For this review, take the finished solid that the model builds, in its own axes (mm). A direction names the side the tool comes from. Coordinates: 2 decimals unless noted, no trailing zeros. Order: outer loops, then holes, each group sorted by start corner. A loop starts at its lowest first (then second) coordinate and runs counter-clockwise, first axis right, second up. Notation, with made-up numbers: (-16, -15) - (39, -15) arc R33 ccw to (39, 20) - close; hole circle Ø9 at (48, 13.5). An arc over 180 degrees is marked (long way). One line per item, written item: value. Start each with the question number.
(1) Consider section C-C on y = 62. Write out the cut boundary in (x, z) (3 decimals), then the cut area to 3 significant figures.
(2) Consider section D-D on x = 34. Write out the cut boundary in (y, z).
(3) For faces 1 (the cylindrical face through (18.37, 87.68, 11.06)), 2 (the flat face through (10, 0, 7)), list the 3-axis set-ups (+Z, -Z, +X, -X, +Y, -Y) from which the entire face can be reached by the end or side of a thin tool; tool diameter is ignored.
(4) Consider section A-A on z = 5. Write out the cut boundary in (x, y).
(5) To check wall thickness, follow line 1 along Y through (x, z) = (55, 5.75); line 2 along Y through (x, z) = (130, 1.5); line 3 along X through (y, z) = (100, 10.5). State the ranges of each line that lie inside material, in increasing order.
(6) Consider section B-B on x = 130. Write out the cut boundary in (y, z).
(7) Clearance check with flat-ended pins moving along their axes: pin 1 (4.5 mm diameter, centred on x = 17, y = 97, fed in from +Z); pin 2 (8 mm diameter, centred on y = 38.5, z = 12, fed in from +X); pin 3 (14 mm diameter, centred on x = 93, y = 100, fed in from +Z); pin 4 (2 mm diameter, centred on x = 67, z = 2, fed in from -Y). State where each tip first meets the part, or that it passes through.
(8) Mouldability with a two-part tool opening along X and no side actions: class faces 3 (the flat face through (61, 113, 0)), 4 (the flat face through (88, 68, 7)), 5 (the flat face through (0, 75, 7)), 6 (the flat face through (25, 95, 7)) as released by +X, released by -X, zero draft, split by the parting line, or undercut.
```python
from build123d import *

# Parameters (mm, degrees)
EXTRUDE_1_DEPTH               = 15
HOLE_WIZARD_M20_1_D           = 17.5
HOLE_WIZARD_M20_1_CSINK_D     = 20.05
HOLE_WIZARD_M20_1_CSINK_ANGLE = 90
SKETCH_5_R                    = 4.5
CUT_EXTRUDE_1_DEPTH           = 220.715725427
SKETCH_6_R                    = 7.5
CUT_EXTRUDE_2_DEPTH           = 8


with BuildPart() as part:
    # 스케치1 → 보스-돌출1 (new body)
    with BuildSketch(Plane.XY):
        Polygon((155, 135), (20, 0), (0, 0), (0, 152), (3, 155), (155, 155), align=None)
    extrude(amount=EXTRUDE_1_DEPTH)

    # M20 나사 구멍1 (through all)
    with Locations(Plane.XY.offset(15)):
        with Locations((62, 93), (55, 62), (93, 100)):
            CounterSinkHole(HOLE_WIZARD_M20_1_D / 2, HOLE_WIZARD_M20_1_CSINK_D / 2, counter_sink_angle=HOLE_WIZARD_M20_1_CSINK_ANGLE)

    # 스케치5 → 컷-돌출1 (cut, through all)
    with BuildSketch(Plane.XY.offset(15)):
        with Locations((60, 135)):
            Circle(SKETCH_5_R)
        with Locations((20, 95)):
            Circle(SKETCH_5_R)
        with Locations((130, 135)):
            Circle(SKETCH_5_R)
        with Locations((20, 25)):
            Circle(SKETCH_5_R)
    extrude(amount=-CUT_EXTRUDE_1_DEPTH, mode=Mode.SUBTRACT)

    # 스케치6 → 컷-돌출2 (cut)
    with BuildSketch(Plane.XY.offset(15)):
        with Locations((20, 95)):
            Circle(SKETCH_6_R)
        with Locations((20, 25)):
            Circle(SKETCH_6_R)
        with Locations((60, 135)):
            Circle(SKETCH_6_R)
        with Locations((130, 135)):
            Circle(SKETCH_6_R)
    extrude(amount=-CUT_EXTRUDE_2_DEPTH, mode=Mode.SUBTRACT)


solid = part.part
```
Geometry check:
1. outline: (0, 0) - (46.25, 0) - (46.25, 13.725) - (44.975, 15) - (0, 15) - close; (63.75, 0) - (82, 0) - (82, 15) - (65.025, 15) - (63.75, 13.725) - close
1. area: 966 mm^2
2. outline: (14, 0) - (155, 0) - (155, 15) - (14, 15) - close
3. face 1: +Z
3. face 2: +Z, -Z, +X, -X, -Y
4. outline: (0, 0) - (20, 0) - (155, 135) - (155, 155) - (3, 155) - (0, 152) - close; hole circle Ø9 at (20, 25); hole circle Ø9 at (20, 95); hole circle Ø17.5 at (55, 62); hole circle Ø17.5 at (62, 93); hole circle Ø9 at (60, 135); hole circle Ø17.5 at (93, 100); hole circle Ø9 at (130, 135)
5. line 1: y = 35 to 53.25, 70.75 to 87.75, 98.25 to 155
5. line 2: y = 110 to 130.5, 139.5 to 155
5. line 3: x = 0 to 14.41, 25.59 to 56.75, 67.25 to 84.25, 101.75 to 120
6. outline: (110, 0) - (130.5, 0) - (130.5, 7) - (127.5, 7) - (127.5, 15) - (110, 15) - close; (139.5, 0) - (155, 0) - (155, 15) - (142.5, 15) - (142.5, 7) - (139.5, 7) - close
7. pin 1: stops at z = 7
7. pin 2: stops at x = 62.5
7. pin 3: passes through
7. pin 4: stops at y = 46
8. face 3: zero draft
8. face 4: released by +X
8. face 5: released by -X
8. face 6: undercut
